Verification items for the finished model (mm, model axes). Face numbers are marked on the shaded views. A direction names the side the tool comes from. Coordinates: 2 decimals unless noted, no trailing zeros. Loops run counter-clockwise (first coordinate to the right, second up) from the corner with the lowest first, then second, coordinate; pieces in that order, holes last.
Q1. Access from +Z, -Z, +X, -X, +Y, -Y to the whole of each face (thin tool, end or side, straight path). Record for the marked faces 1, 2 and 3.
Q2. Mould release check, pull along Z, two halves, no side actions. Record for the marked faces 4, 5 and 6: +Z half, -Z half, draft (parallel to the pull), parting line (faces both ways), or undercut.
Q3. Sectioned sample at C-C (x = 35). Count the separate pieces of the cut face and the enclosed holes in it, then the cut area to 3 significant figures.
Q4. Material ranges on probe 1 along X at (y, z) = (75, -43); probe 2 along Y at (x, z) = (35, -9.5); probe 3 along Z at (x, y) = (43, 5.5), recorded low to high.
Q5. Go/stop test with flat-tipped pins: P1, Ø6, axis at x = 35, y = 75, coming from the -Z side; P2, Ø3, axis at x = 7, z = -5, coming from the -Y side; P3, Ø8, axis at x = 6, y = 46.5, coming from the -Z side. Record where each tip stops, or that it passes through.
Q6. Sectioned sample at A-A (y = 75). Enter the section's corners in (x, z), then the cut area to 3 significant figures.
Q7. Sectioned sample at B-B (z = -44.5). Enter the section's corners in (x, y), then the cut area to 3 significant figures.
Autodesk Inventor part; units mm, degrees
ref_plane "YZ Plane" through (0, 0, 0) normal (1, 0, 0) x (0, 1, 0)
ref_plane "XZ Plane" through (0, 0, 0) normal (0, 1, 0) x (-1, 0, 0)
ref_plane "XY Plane" through (0, 0, 0) normal (0, 0, 1) x (1, 0, 0)
sketch "Sketch1" plane through (0, 0, 0) normal (1, 0, 0) x (0, 1, 0)
  ellipse E0 centre (0, -25) end of major axis (45, -25) minor radius 12.5 (0, -37.5) -> (0, -12.5) ccw
  ellipse E1 centre (0, -25) end of major axis (120, -25) minor radius 25 (0, -50) -> (0, 0) ccw
  line L0 (65, -3.9852) -> (65, -46.0148)
  line L1 (0, -37.5) -> (0, -50)
  line L2 (0, -12.5) -> (0, 0)
  point P0 (0, -43.75)
  point P1 (0, -6.25)
  dimension "d23" = 45
  dimension "d25" = 120
  dimension "d18" = 50
  dimension "d22" = 25
  dimension "d24" = 65
extrude "Extrusion1" add sketch "Sketch1" along normal blind 50 contours E0 L2 E1 L0 L1
sketch "Sketch3" plane through (0, 65, -3.9852) normal (0, 1, 0) x (1, 0, 0)
  line L0 (0, 42.0297) -> (0, 0)
  line L1 (0, 0) -> (50, 0)
  line L2 (50, 42.0297) -> (50, 0)
  line L3 (0, 42.0297) -> (50, 42.0297)
  line L4 (0, 33.5148) -> (0, 8.5148)
  line L5 (50, 0) -> (0, 0)
  line L6 (0, 0) -> (0, 8.5148)
  line L7 (0, 8.5148) -> (50, 8.5148)
  line L8 (50, 8.5148) -> (50, 0)
  line L9 (0, 42.0297) -> (50, 42.0297)
  line L10 (50, 42.0297) -> (50, 33.5148)
  line L11 (50, 33.5148) -> (0, 33.5148)
  line L12 (0, 33.5148) -> (0, 42.0297)
  point P0 (0, -3.9852)
  point P1 (0, 33.5148)
  dimension "d26" = 25
  dimension "d27" = 8.5148
  dimension "d28" = 8.5148
extrude "Extrusion3" add sketch "Sketch3" along normal blind 20 contours L3 L2 L11 L0 | L7 L2 L1 L0
sketch "Sketch4" plane through (50, 65, -46.0148) normal (0, 0, -1) x (-1, 0, 0)
  line L0 (50, 0) -> (0, 0)
  line L1 (50, 0) -> (50, 20)
  line L2 (0, 20) -> (50, 20)
  line L3 (0, 0) -> (0, 20)
  line L4 (0, 0) -> (0, 20)
  line L5 (0, 10) -> (50, 10)
  circle A0 centre (15, 10) radius 2.25
  circle A1 centre (35, 10) radius 2.25
  point P0 (50, -65)
  dimension "d31" = 4.5
  dimension "d32" = 4.5
  dimension "d33" = 20
  dimension "d34" = 15
  dimension "d35" = 15
extrude "Extrusion4" cut sketch "Sketch4" against normal through all contours A1 L5 | L5 A1 | A0 L5 | L5 A0
sketch "Sketch5" plane through (0, 0, -12.5) normal (0, -1, 0) x (1, 0, 0)
  line L0 (0, 12.5) -> (0, 0)
  line L1 (0, 0) -> (50, 0)
  line L2 (50, 12.5) -> (50, 0)
  line L3 (0, 12.5) -> (50, 12.5)
  line L4 (0, -25) -> (0, -37.5)
  line L5 (0, -37.5) -> (50, -37.5)
  line L6 (50, -25) -> (50, -37.5)
  line L7 (0, -25) -> (50, -25)
  line L8 (50, 8.5148) -> (50, 12.5)
  line L9 (0, -25) -> (0, -37.5)
  line L10 (50, 12.5) -> (0, -37.5)
  line L11 (5.7, 6.8) -> (44.3, 6.8)
  line L12 (44.3, 6.8) -> (44.3, -31.8)
  line L13 (44.3, -31.8) -> (5.7, -31.8)
  line L14 (5.7, -31.8) -> (5.7, 6.8)
  line L15 (5.7, 6.8) -> (44.3, -31.8) construction
  line L16 (44.3, 6.8) -> (5.7, -31.8) construction
  line L17 (44.3, 3.3) -> (41.2689, 5.05)
  line L18 (41.2689, 5.05) -> (41.2689, 8.55)
  line L19 (41.2689, 8.55) -> (44.3, 10.3)
  line L20 (44.3, 10.3) -> (47.3311, 8.55)
  line L21 (47.3311, 8.55) -> (47.3311, 5.05)
  line L22 (47.3311, 5.05) -> (44.3, 3.3)
  line L23 (41.2689, -33.55) -> (41.2689, -30.05)
  line L24 (41.2689, -30.05) -> (44.3, -28.3)
  line L25 (44.3, -28.3) -> (47.3311, -30.05)
  line L26 (47.3311, -30.05) -> (47.3311, -33.55)
  line L27 (47.3311, -33.55) -> (44.3, -35.3)
  line L28 (44.3, -35.3) -> (41.2689, -33.55)
  line L29 (8.7311, -30.05) -> (8.7311, -33.55)
  line L30 (8.7311, -33.55) -> (5.7, -35.3)
  line L31 (5.7, -35.3) -> (2.6689, -33.55)
  line L32 (2.6689, -33.55) -> (2.6689, -30.05)
  line L33 (2.6689, -30.05) -> (5.7, -28.3)
  line L34 (5.7, -28.3) -> (8.7311, -30.05)
  line L35 (8.7311, 8.55) -> (8.7311, 5.05)
  line L36 (8.7311, 5.05) -> (5.7, 3.3)
  line L37 (5.7, 3.3) -> (2.6689, 5.05)
  line L38 (2.6689, 5.05) -> (2.6689, 8.55)
  line L39 (2.6689, 8.55) -> (5.7, 10.3)
  line L40 (5.7, 10.3) -> (8.7311, 8.55)
  point P0 (25, -12.5)
  dimension "d38" = 38.6
  dimension "d39" = 38.6
  dimension "d40" = 7
  dimension "d41" = 7
  dimension "d42" = 7
  dimension "d43" = 7
extrude "Extrusion5" cut sketch "Sketch5" against normal blind 10 contours L20 L21 L22 L12 L10 | L10 L11 L18 L19 L20 | L37 L38 L39 L40 L35 L11 L14 | L14 L11 L35 L36 | L12 L17 L10 | L10 L17 L18 L11 | L34 L10 L14 | L14 L10 L31 L32 L33 | L34 L29 L13 L10 | L13 L29 L30 L31 L10 | L25 L26 L27 L28 L23 L13 L12 | L12 L13 L23 L24
equation "\"d27\" = d28"
properties part number "Arch" material "ABS Plastic"
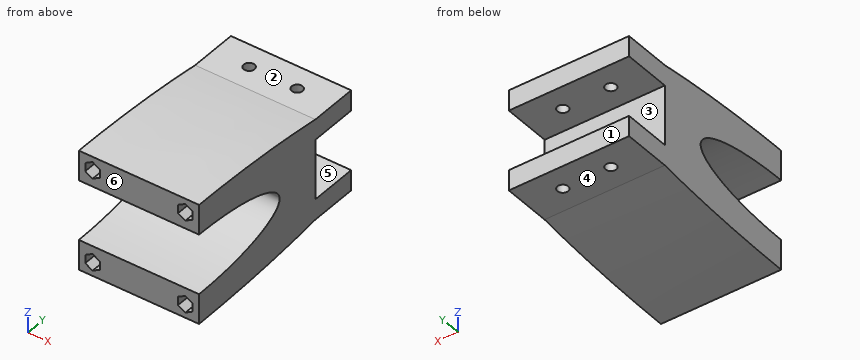
Geometry check:
1. face 1: +Z, -Z, +X, -X, +Y
1. face 2: +Z, +X, -X, +Y
1. face 3: +X, -X, +Y
2. face 4: -Z half
2. face 5: undercut
2. face 6: draft
3. separate pieces: 3
3. enclosed holes: 0
3. area: 2,460 mm2
4. probe 1: x = 0 to 12.75, 17.25 to 32.75, 37.25 to 50
4. probe 2: y = 0 to 72.75, 77.25 to 85
4. probe 3: z = -49.97 to -47.05, -41.55 to -37.41, -12.59 to -8.45, -2.95 to -0.03
5. P1: stops at z = -46.01
5. P2: stops at y = 10
5. P3: stops at z = -48.38
6. outline: (0, -46.01) - (12.75, -46.01) - (12.75, -37.5) - (0, -37.5) - close; (0, -12.5) - (12.75, -12.5) - (12.75, -3.99) - (0, -3.99) - close; (17.25, -46.01) - (32.75, -46.01) - (32.75, -37.5) - (17.25, -37.5) - close; (17.25, -12.5) - (32.75, -12.5) - (32.75, -3.99) - (17.25, -3.99) - close; (37.25, -46.01) - (50, -46.01) - (50, -37.5) - (37.25, -37.5) - close; (37.25, -12.5) - (50, -12.5) - (50, -3.99) - (37.25, -3.99) - close
6. area: 698 mm2
7. outline: (0, 0) - (2.67, 0) - (2.67, 10) - (8.73, 10) - (8.73, 0) - (41.27, 0) - (41.27, 10) - (47.33, 10) - (47.33, 0) - (50, 0) - (50, 85) - (0, 85) - close; hole circle Ø4.5 at (15, 75); hole circle Ø4.5 at (35, 75)
7. area: 4,100 mm2
